Study the drawing (mm; zero at the part's minimum x, y, z) and answer. Coordinates: 2 decimals unless noted, no trailing zeros. Order: outer loops, then holes, each group sorted by start corner. A loop starts at its lowest first (then second) coordinate and runs counter-clockwise, first axis right, second up. Notation, with made-up numbers: (-2.5, 28.25) - (47.5, 28.25) arc R17 ccw to (47.5, 50.25) - close; hole circle Ø2 at (37, 49.5). An arc over 180 degrees is marked (long way). Write item = value, one per line.
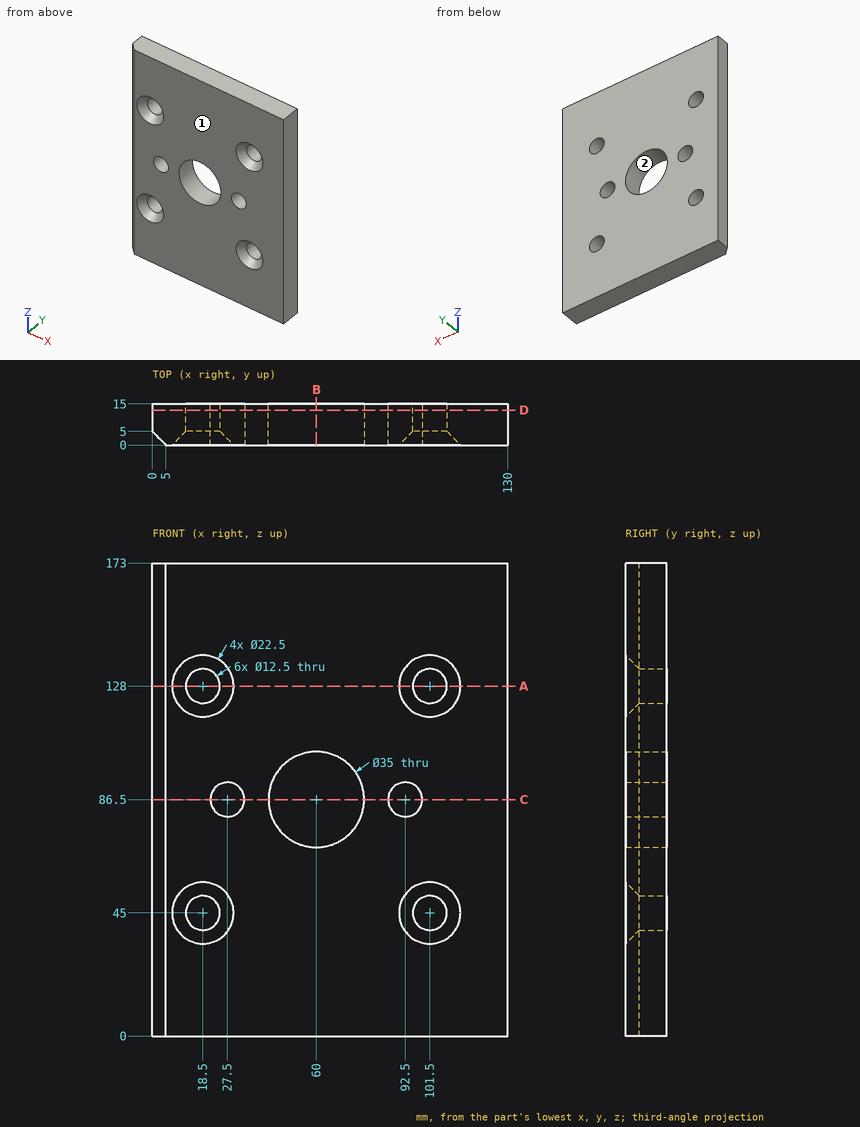
1) The part is cut by section D-D (y = 12.75). Determine the outline of the cut face in (x, z).
Returned:
outline = (0, 0) - (130, 0) - (130, 173) - (0, 173) - close; hole circle Ø12.5 at (18.5, 45); hole circle Ø12.5 at (18.5, 128); hole circle Ø12.5 at (27.5, 86.5); hole circle Ø35 at (60, 86.5); hole circle Ø12.5 at (92.5, 86.5); hole circle Ø12.5 at (101.5, 45); hole circle Ø12.5 at (101.5, 128)
2) Straight lines are drawn through the part: line 1 along Z through (x, y) = (101.5, 12); line 2 along Z through (x, y) = (23.5, 14); line 3 along X through (y, z) = (12.5, 41). For each, find the intervals that lie inside material, in ascending order. Write a range as from..to.
Returned:
line_1 = 0..38.75, 51.25..121.75, 134.25..173
line_2 = 0..41.25, 48.75..81.7, 91.3..124.25, 131.75..173
line_3 = 0..13.7, 23.3..96.7, 106.3..130
3) The part is cut by section A-A (z = 128). Determine the outline of the cut face in (x, y), and give its area (3 significant figures).
Returned:
outline = (0, 5) - (5, 0) - (7.25, 0) - (12.25, 5) - (12.25, 15) - (0, 15) - close; (24.75, 5) - (29.75, 0) - (90.25, 0) - (95.25, 5) - (95.25, 15) - (24.75, 15) - close; (107.75, 5) - (112.75, 0) - (130, 0) - (130, 15) - (107.75, 15) - close
area = 1,510 mm^2
4) Determine the mould class of the marked faces 1 and 2 for opening direction Z: pulls with the +Z half, pulls with the -Z half, needs draft (parallel to the pull), parting line crosses it, or undercut.
Returned:
face_1 = needs draft
face_2 = undercut
5) The part is cut by section B-B (x = 60). Determine the outline of the cut face in (y, z), and give its area (3 significant figures).
Returned:
outline = (0, 0) - (15, 0) - (15, 69) - (0, 69) - close; (0, 104) - (15, 104) - (15, 173) - (0, 173) - close
area = 2,070 mm^2
6) The part is cut by section C-C (z = 86.5). Determine the outline of the cut face in (x, y).
Returned:
outline = (0, 5) - (5, 0) - (21.25, 0) - (21.25, 15) - (0, 15) - close; (33.75, 0) - (42.5, 0) - (42.5, 15) - (33.75, 15) - close; (77.5, 0) - (86.25, 0) - (86.25, 15) - (77.5, 15) - close; (98.75, 0) - (130, 0) - (130, 15) - (98.75, 15) - close
